Study the drawing (mm; zero at the part's minimum x, y, z) and answer. Round coordinates to 2 decimals unless told otherwise and drop trailing zeros. Order: outer loops, then holes, each group sorted by start corner. A loop starts at its lowest first (then second) coordinate and runs counter-clockwise, first axis right, second up. Notation, with made-up numbers: M 20,73 L 30,73 A31 ccw 30,97 Z; hole C 24.5,49.25 d11. An arc over 180 degrees is marked long. Put each result on its own line as item: value. Start each with the question number.
1. The part is cut by section A-A (y = 0.8). Give the vertices of the cut face in (x, z).
2. The part is cut by section B-B (z = 10). Give the vertices of the cut face in (x, y), then the cut area to 3 significant figures.
3. The part is cut by section C-C (x = 13.5). Give the vertices of the cut face in (y, z), then the cut area to 3 significant figures.
4. Each of these flat-tipped pins is pushed along its axis until it touches: pin 1 Ø2 at (y, z) = (2, 3.5) entering from -X; pin 2 Ø1.2 at (x, y) = (28.5, 2) entering from -Z; pin 3 Ø2 at (y, z) = (1.5, 106.5) entering from +X; pin 4 Ø2 at (x, z) = (24, 88.5) entering from -Y. Where does it stop, or does it pass through?
5. Consider line 1 (Z direction, x = 5.5, y = 2.45); line 2 (X direction, y = 1.4, z = 102); line 3 (Z direction, x = 29, y = 1.9). Determine where each line is inside the solid, lowest interval first.
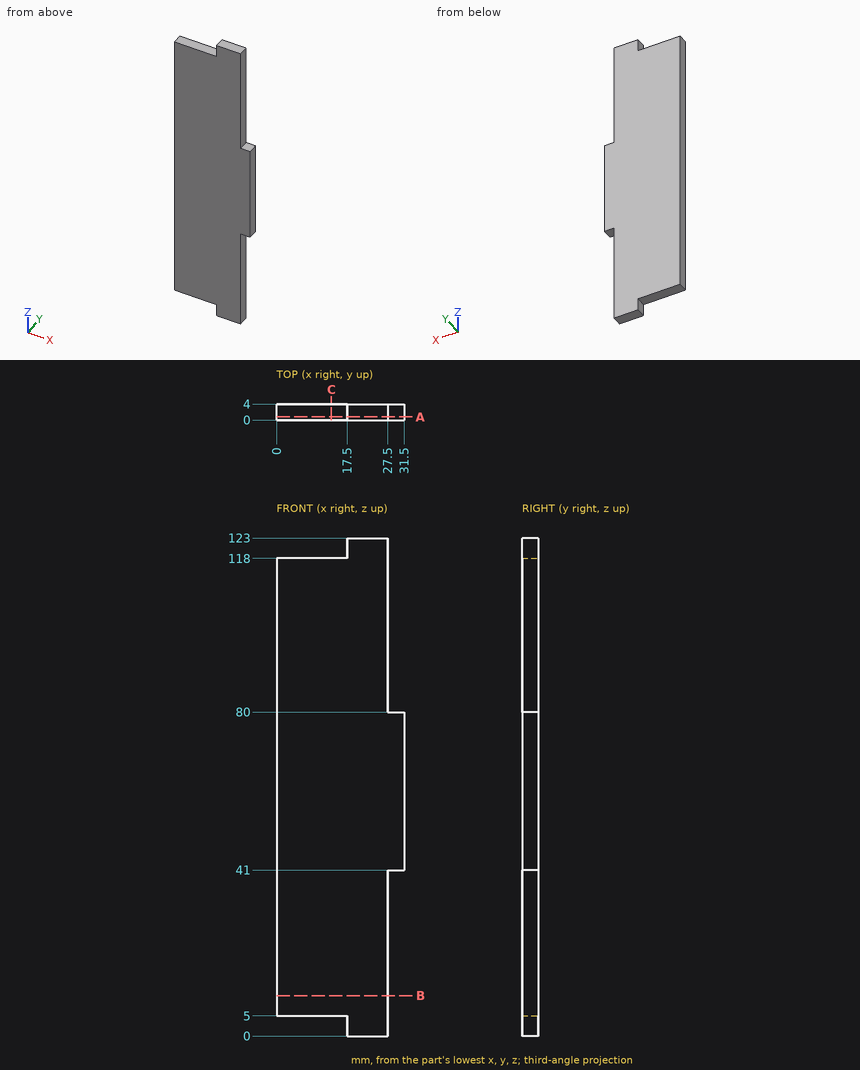
Resolved:
1. outline: M 0,5 L 17.5,5 L 17.5,0 L 27.5,0 L 27.5,41 L 31.5,41 L 31.5,80 L 27.5,80 L 27.5,123 L 17.5,123 L 17.5,118 L 0,118 Z
2. outline: M 0,0 L 27.5,0 L 27.5,4 L 0,4 Z
2. area: 110 mm2
3. outline: M 0,5 L 4,5 L 4,118 L 0,118 Z
3. area: 452 mm2
4. pin 1: x = 17.5
4. pin 2: z = 41
4. pin 3: x = 27.5
4. pin 4: y = 0
5. line 1: 5 to 118
5. line 2: 0 to 27.5
5. line 3: 41 to 80
